```python
from build123d import *

# Parameters (mm, degrees)
SKETCH_1_R               = 4
EXTRUDE_1_DEPTH          = 20
CUT_EXTRUDE_1_DEPTH      = 138.563388298
CUT_EXTRUDE_1_DEPTH_BACK = 138.563388298
SKETCH_2_W               = 23
SKETCH_2_H               = 25


with BuildPart() as part:
    # 草图1 → 凸台-拉伸1 (new, symmetric)
    with BuildSketch(Plane(origin=(0, 0, 0), x_dir=(1, 0, 0), z_dir=(0, 1, 0))):
        with BuildLine():
            Line((-7.673488412, -2.262205913), (5.894069743, -48.283878695))
            ThreePointArc((5.894069743, -48.283878695), (7.695788374, -50.874334744), (10.69, -51.87))
            Line((10.69, -51.87), (38.585207042, -51.87))
            ThreePointArc((38.585207042, -51.87), (70.04, -38.09), (101.494792958, -51.87))
            Line((101.494792958, -51.87), (120.83, -51.87))
            ThreePointArc((120.83, -51.87), (124.79417955, -49.917175823), (125.661820833, -45.584112198))
            Line((125.661820833, -45.584112198), (124.011820833, -39.384112198))
            ThreePointArc((124.011820833, -39.384112198), (122.875351803, -37.301858813), (120.907082582, -35.97775259))
            Line((120.907082582, -35.97775259), (2.763332132, 7.507595856))
            ThreePointArc((2.763332132, 7.507595856), (-5.467144165, 5.840405352), (-7.673488412, -2.262205913))
        make_face()
        with Locations(Location((0, 0, 0), (0, 0, 270))):
            Circle(SKETCH_1_R, mode=Mode.SUBTRACT)
        with Locations(Location((7.33, -24.87, 0), (0, 0, 270))):
            Circle(SKETCH_1_R, mode=Mode.SUBTRACT)
    extrude(amount=EXTRUDE_1_DEPTH, both=True)

    # 草图2 → 切除-拉伸1 (cut, two sides: drawn at the far end of the back side and taken through both)
    with BuildSketch(Plane.XY.offset(-CUT_EXTRUDE_1_DEPTH_BACK)):
        with Locations((3.5, 0)):
            Rectangle(SKETCH_2_W, SKETCH_2_H)
    extrude(amount=CUT_EXTRUDE_1_DEPTH + CUT_EXTRUDE_1_DEPTH_BACK, mode=Mode.SUBTRACT)


solid = part.part
```
The model under review builds one solid part; all positions refer to its coordinate system, in mm. A direction names the side the tool comes from. Coordinates: 2 decimals unless noted, no trailing zeros. Order: outer loops, then holes, each group sorted by start corner. A loop starts at its lowest first (then second) coordinate and runs counter-clockwise, first axis right, second up. Notation, with made-up numbers: (23.25, 37.25) -> (46.25, 37.25) arc R13 ccw to (46.25, 41.25) -> close; hole circle Ø7 at (54, 47.5). An arc over 180 degrees is marked (long way). Answer in a Markdown table with one row per item. Add a question column.
Item 1: We need section C-C on z = 24.87. Write out the cut boundary in (x, y).
Item 2: Mouldability with a two-part tool opening along Z and no side actions: class faces 1 (the flat face through (6, -12.5, 15)), 2 (the flat face through (-0.985, -16.197, 24.951)), 3 (the cylindrical face through (-5.4, -16.2, -5.9)), 4 (the cylindrical face through (5.798, 16.197, 28.565)) as +Z half, -Z half, draft (parallel to the pull), parting line (faces both ways), or undercut.
Item 3: We need section B-B on y = -15.5. Write out the cut boundary in (x, z), plus the area to 3 significant figures.
Item 4: Clearance check with flat-ended pins moving along their axes: pin 1 (1.5 mm diameter, centred on y = -6.5, z = 12.5, fed in from -X); pin 2 (6 mm diameter, centred on x = 30.5, y = -1.5, fed in from -Z); pin 3 (8 mm diameter, centred on x = 102.5, z = 26.5, fed in from +Y); pin 4 (5 mm diameter, centred on x = 106, y = -2, fed in from -Z). State where each tip first meets the part, or that it passes through.
Item 5: We need section D-D on y = -1.5. Write out the cut boundary in (x, z), plus the area to 3 significant figures.
Item 6: We need section A-A on x = 7.33. Write out the cut boundary in (y, z).
Item 7: To check wall thickness, follow probe 1 along Y at (x, z) = (11, 13.5); probe 2 along X at (y, z) = (-3.5, 46); probe 3 along Z at (x, y) = (71.5, 5.5). State the ranges of each line that lie inside material, in increasing order.
Item 8: Machinability: for faces 5 (the flat face through (-0.985, 16.303, 24.951)), 6 (the flat face through (6, 12.5, 15)), which of the approach directions +Z, -Z, +X, -X, +Y, -Y give a long, thin tool a straight path to every point of the face, cutting with its end or side? Answer none if there is none.
Final values:
| question | item | result |
|---|---|---|
| 1 | outline | (-1.01, -20) -> (3.33, -20) -> (3.33, -12.5) -> (-1.01, -12.5) -> close; (-1.01, 12.5) -> (3.33, 12.5) -> (3.33, 20) -> (-1.01, 20) -> close; (11.33, -20) -> (90.73, -20) -> (90.73, 20) -> (11.33, 20) -> (11.33, 12.5) -> (15, 12.5) -> (15, -12.5) -> (11.33, -12.5) -> close |
| 2 | face 1 | draft |
| 2 | face 2 | +Z half |
| 2 | face 3 | parting line |
| 2 | face 4 | undercut |
| 3 | outline | (-7.67, 2.26) arc R8 ccw to (2.76, -7.51) -> (120.91, 35.98) arc R5 ccw to (124.01, 39.38) -> (125.66, 45.58) arc R5 ccw to (120.83, 51.87) -> (101.49, 51.87) arc R42.79 cw to (38.59, 51.87) -> (10.69, 51.87) arc R5 ccw to (5.89, 48.28) -> close; hole circle Ø8 at (0, 0); hole circle Ø8 at (7.33, 24.87) |
| 3 | area | 4,050 mm2 |
| 4 | pin 1 | stops at x = 15 |
| 4 | pin 2 | stops at z = 1.6 |
| 4 | pin 3 | stops at y = 20 |
| 4 | pin 4 | stops at z = 29.57 |
| 5 | outline | (15, -3) -> (120.91, 35.98) arc R5 ccw to (124.01, 39.38) -> (125.66, 45.58) arc R5 ccw to (120.83, 51.87) -> (101.49, 51.87) arc R42.79 cw to (38.59, 51.87) -> (15, 51.87) -> close |
| 5 | area | 3,200 mm2 |
| 6 | outline | (-20, -5.83) -> (-12.5, -5.83) -> (-12.5, 20.87) -> (-20, 20.87) -> close; (-20, 28.87) -> (-12.5, 28.87) -> (-12.5, 50.57) -> (-20, 50.57) -> close; (12.5, -5.83) -> (20, -5.83) -> (20, 20.87) -> (12.5, 20.87) -> close; (12.5, 28.87) -> (20, 28.87) -> (20, 50.57) -> (12.5, 50.57) -> close |
| 7 | probe 1 | y = -20 to -12.5, 12.5 to 20 |
| 7 | probe 2 | x = 15 to 45.25, 94.83 to 125.75 |
| 7 | probe 3 | z = 17.79 to 38.11 |
| 8 | face 5 | +Z, -X, +Y, -Y |
| 8 | face 6 | +Z, -Z, -X |
